```python
from build123d import *

# Parameters (mm, degrees)
SKETCH_W  = 140
SKETCH_H  = 140
SKETCH_R  = 21
PAD_DEPTH = 4


with BuildPart() as part:
    # Sketch → Pad (new body)
    with BuildSketch(Plane.XZ):
        Rectangle(SKETCH_W, SKETCH_H)
        Circle(SKETCH_R, mode=Mode.SUBTRACT)
        Polygon((-40, 19), (-21.813467, 50.5), (-58.186533, 50.5), align=None, mode=Mode.SUBTRACT)
        Polygon((40, -19), (21.813467, -50.5), (58.186533, -50.5), align=None, mode=Mode.SUBTRACT)
        Polygon((27.65651, 23.010643), (52.34349, 23.010643), (59.972187, 46.489357), (40, 61), (20.027813, 46.489357), align=None, mode=Mode.SUBTRACT)
        Polygon((-21.813467, -29.5), (-40, -19), (-58.186533, -29.5), (-58.186533, -50.5), (-40, -61), (-21.813467, -50.5), align=None, mode=Mode.SUBTRACT)
    extrude(amount=PAD_DEPTH)


solid = part.part
```
Can you work these out from the model? Positions are in its coordinate system, mm. A direction names the side the tool comes from. Round coordinates to 2 decimals unless told otherwise and drop trailing zeros. Loops run counter-clockwise (first coordinate to the right, second up) from the corner with the lowest first, then second, coordinate; pieces in that order, holes last.
Item 1: Suppose I cut it at C-C, the plane y = -0.65. Write out the boundary of the cut face in (x, z), then the cut area to 3 significant figures.
Item 2: Which directions (+Z, -Z, +X, -X, +Y, -Y) give clear straight access to the entire face, cutting with the end or side of a thin tool? Please do faces 4 (the flat face through (-17, 0, 17)), 5 (the flat face through (56.104, -1.972, 34.586)).
Item 3: If we mould it in two halves opening along X, with no side actions, what happens to faces 1 (the cylindrical face through (20.03, -1.97, 6.31)), 2 (the flat face through (70, -2, -1)), 3 (the flat face through (-70, -2, -1))? For each: +X half, -X half, draft (parallel to the pull), parting line (faces both ways), or undercut.
Item 4: Please list where these lines run through material, in increasing order: L1, parallel to Z at x = 0, y = -3.05; L2, parallel to X at y = -3.75, z = -31.5; L3, parallel to X at y = -1.2, z = -45.5.
Item 5: Suppose I cut it at A-A, the plane x = 0. Write out the boundary of the cut face in (y, z), then the cut area to 3 significant figures.
Item 6: Suppose I cut it at B-B, the plane z = 0. Write out the boundary of the cut face in (x, y), then the cut area to 3 significant figures.
Item 7: Suppose I cut it at D-D, the plane x = -34.5. Write out the boundary of the cut face in (y, z), then the cut area to 3 significant figures.
Reported:
1. outline: (-70, -70) - (70, -70) - (70, 70) - (-70, 70) - close; hole (-58.19, -50.5) - (-40, -61) - (-21.81, -50.5) - (-21.81, -29.5) - (-40, -19) - (-58.19, -29.5) - close; hole (-58.19, 50.5) - (-40, 19) - (-21.81, 50.5) - close; hole circle Ø42 at (0, 0); hole (20.03, 46.49) - (27.66, 23.01) - (52.34, 23.01) - (59.97, 46.49) - (40, 61) - close; hole (21.81, -50.5) - (58.19, -50.5) - (40, -19) - close
1. area: 14,900 mm2
2. face 4: +Z, -Z, +X, -X, +Y
2. face 5: +Y, -Y
3. face 1: undercut
3. face 2: +X half
3. face 3: -X half
4. L1: z = -70 to -21, 21 to 70
4. L2: x = -70 to -58.19, -21.81 to 32.78, 47.22 to 70
4. L3: x = -70 to -58.19, -21.81 to 24.7, 55.3 to 70
5. outline: (-4, -70) - (0, -70) - (0, -21) - (-4, -21) - close; (-4, 21) - (0, 21) - (0, 70) - (-4, 70) - close
5. area: 392 mm2
6. outline: (-70, -4) - (-21, -4) - (-21, 0) - (-70, 0) - close; (21, -4) - (70, -4) - (70, 0) - (21, 0) - close
6. area: 392 mm2
7. outline: (-4, -70) - (0, -70) - (0, -57.82) - (-4, -57.82) - close; (-4, -22.18) - (0, -22.18) - (0, 28.53) - (-4, 28.53) - close; (-4, 50.5) - (0, 50.5) - (0, 70) - (-4, 70) - close
7. area: 330 mm2
